```python
from build123d import *

# Parameters (mm, degrees)
BOSS_EXTRUDE8_DEPTH = 10
SKETCH8_R           = 50
BOSS_EXTRUDE9_DEPTH = 25
SKETCH9_R           = 5
CUT_EXTRUDE8_DEPTH  = 5
FILLET1_R           = 10


with BuildPart() as part:
    # Sketch1 → Boss-Extrude8 (new body)
    with BuildSketch(Plane(origin=(0, 0, 0), x_dir=(1, 0, 0), z_dir=(0, 1, 0))):
        with BuildLine():
            ThreePointArc((50, 0), (35.355339059, 35.355339059), (0, 50))
            Line((0, 50), (0, -50))
            ThreePointArc((0, -50), (35.355339059, -35.355339059), (50, 0))
        make_face()
        with BuildLine():
            Line((0, -50), (0, 50))
            ThreePointArc((0, 50), (-50, 0), (0, -50))
        make_face()
        with BuildLine():
            ThreePointArc((0, -50), (-50, 0), (0, 50))
            Line((0, 50), (-130, 50))
            Line((-130, 50), (-130, -50))
            Line((-130, -50), (0, -50))
        make_face()
    extrude(amount=BOSS_EXTRUDE8_DEPTH)

    # Sketch8 → Boss-Extrude9 (add)
    with BuildSketch(Plane(origin=(0, 10, 0), x_dir=(1, 0, 0), z_dir=(0, 1, 0))):
        with Locations(Location((0, 0, 0), (0, 0, 270))):
            Circle(SKETCH8_R)
    extrude(amount=BOSS_EXTRUDE9_DEPTH)

    # Sketch9 → Cut-Extrude8 (cut)
    with BuildSketch(Plane.XZ):
        with Locations(Location((-15, 40, 0), (0, 0, 270))):
            Circle(SKETCH9_R)
        with Locations(Location((-15, -40, 0), (0, 0, 270))):
            Circle(SKETCH9_R)
        with Locations(Location((-115, -40, 0), (0, 0, 270))):
            Circle(SKETCH9_R)
        with Locations(Location((-115, 40, 0), (0, 0, 270))):
            Circle(SKETCH9_R)
    extrude(amount=-CUT_EXTRUDE8_DEPTH, mode=Mode.SUBTRACT)

    # Fillet1
    fillet1_edges = [part.edges().sort_by_distance(p)[0] for p in [
        (-130, 5, 50),
        (-130, 5, -50),
    ]]
    fillet(fillet1_edges, radius=FILLET1_R)


solid = part.part
```
Input: part model. Units: mm. Frame: model coordinates. A direction names the side the tool comes from. Give positions to 0.01 mm unless a question says otherwise; leave off trailing zeros. Loops run counter-clockwise (first coordinate to the right, second up) from the corner with the lowest first, then second, coordinate; pieces in that order, holes last. Notation, with made-up numbers: M 70,49.25 L 129,49.25 A19 ccw 129,62.25 Z; hole C 16,56 d3. An arc over 180 degrees is marked long. Answer as CSV lines item,"result". Start each with the question number.
1. Pin query (flat end, axial travel): P1, Ø10, axis at x = 25.5, y = 6.5, coming from the +Z side; P2, Ø3, axis at x = -14, z = 42, coming from the -Y side; P3, Ø1.5, axis at y = 25, z = -19.5, coming from the +X side. Return the tip coordinate at first contact, or that it passes through.
2. Section C-C on y = 17.5. Return loops of the section in (x, z), plus the area to 3 significant figures.
3. Reachability of faces 4 (the face through (1, 35, -1)), 5 (the face through (-15, 5, 40)) from +Z, -Z, +X, -X, +Y, -Y: full face, straight path, thin tool, end or side. Return the list, or none.
4. Section B-B on x = -15. Return loops of the section in (y, z).
5. Line query: L1, parallel to X at y = 3.05, z = -40; L2, parallel to Y at x = -117, z = -44.5; L3, parallel to Y at x = -71, z = 21.5. Output: solid intervals per line, ascending.
6. Section D-D on z = 19. Return loops of the section in (x, y).
7. Section A-A on z = -30. Return loops of the section in (x, y), plus the area to 3 significant figures.
8. Pull-direction query (X, two-part tool) for faces 1 (the face through (-15, 5, -40)), 2 (the face through (-126.99, 5.07, 47.15)), 3 (the face through (-61, 5, 50)); classes: released by +X, released by -X, zero draft, split by the parting line, or undercut.
Computed values:
1,P1,"stops at z = 45.6"
1,P2,"stops at y = 5"
1,P3,"stops at x = 46.35"
2,outline,"C 0,0 d100"
2,area,"7,850 mm²"
3,face 4,"+Z, -Z, +X, -X, +Y"
3,face 5,"-Y"
4,outline,"M 0,-50 L 10,-50 L 10,-47.7 L 35,-47.7 L 35,47.7 L 10,47.7 L 10,50 L 0,50 L 0,45 L 5,45 L 5,35 L 0,35 L 0,-35 L 5,-35 L 5,-45 L 0,-45 Z"
5,L1,"x = -130 to -120, -110 to -20, -10 to 30"
5,L2,"y = 5 to 10"
5,L3,"y = 0 to 10"
6,outline,"M -130,0 L 46.25,0 L 46.25,35 L -46.25,35 L -46.25,10 L -130,10 Z"
7,outline,"M -130,0 L 40,0 L 40,35 L -40,35 L -40,10 L -130,10 Z"
7,area,"3,700 mm²"
8,face 1,"undercut"
8,face 2,"released by -X"
8,face 3,"zero draft"
